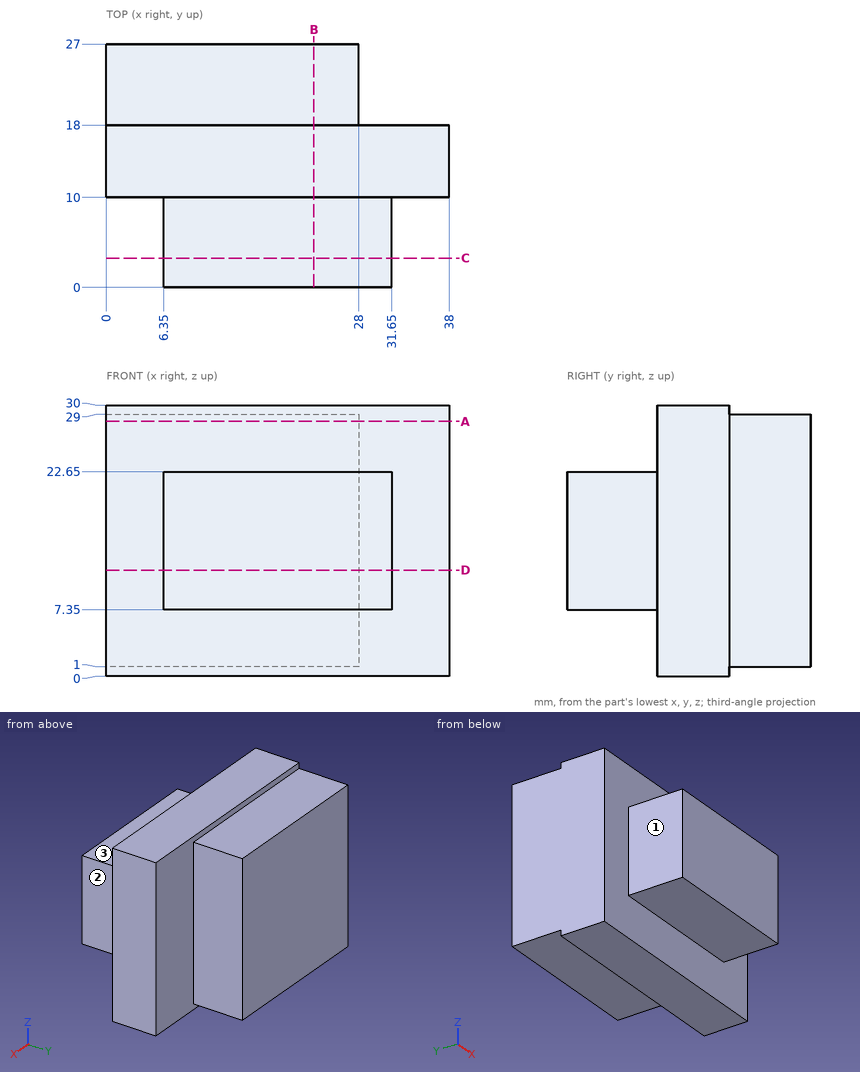
Verification items for this drawing (mm, ordinates from the low corner). A direction names the side the tool comes from. Coordinates: 2 decimals unless noted, no trailing zeros. Order: outer loops, then holes, each group sorted by start corner. A loop starts at its lowest first (then second) coordinate and runs counter-clockwise, first axis right, second up. Notation, with made-up numbers: (-13.5, 35.5) -> (8.5, 35.5) arc R19 ccw to (8.5, 60.5) -> close; hole circle Ø4 at (18, 22.25). An arc over 180 degrees is marked (long way). Answer as CSV lines item,"result". Start each with the question number.
1) Gauge pin test, flat ends, axial feed: pin 1 Ø8 at (y, z) = (3.5, 14) entering from -X; pin 2 Ø5 at (x, y) = (9.5, 23) entering from +Z; pin 3 Ø2 at (x, z) = (19, 4) entering from -Y. Record the tip position at first contact, or that the pin passes through.
2) Cross-section at C-C, the plane y = 3.25. Record the boundary of the cut face in (x, z).
3) Cross-section at B-B, the plane x = 23. Record the boundary of the cut face in (y, z).
4) Cross-section at A-A, the plane z = 28.25. Record the boundary of the cut face in (x, y), then the cut area to 3 significant figures.
5) Cross-section at D-D, the plane z = 11.75. Record the boundary of the cut face in (x, y).
6) Set-up check for the marked faces 1, 2 and 3: record each of +Z, -Z, +X, -X, +Y, -Y from which the full face is reachable in a straight line by a thin tool's end or side.
7) Material ranges on L1, parallel to Y at x = 30, z = 24.75; L2, parallel to Y at x = 15, z = 4.5; L3, parallel to Z at x = 6.5, y = 7.25, recorded low to high. Write a range as [from, to].
Conclusion:
1,pin 1,"stops at x = 6.35"
1,pin 2,"stops at z = 29"
1,pin 3,"stops at y = 10"
2,outline,"(6.35, 7.35) -> (31.65, 7.35) -> (31.65, 22.65) -> (6.35, 22.65) -> close"
3,outline,"(0, 7.35) -> (10, 7.35) -> (10, 0) -> (18, 0) -> (18, 1) -> (27, 1) -> (27, 29) -> (18, 29) -> (18, 30) -> (10, 30) -> (10, 22.65) -> (0, 22.65) -> close"
4,outline,"(0, 10) -> (38, 10) -> (38, 18) -> (28, 18) -> (28, 27) -> (0, 27) -> close"
4,area,"556 mm²"
5,outline,"(0, 10) -> (6.35, 10) -> (6.35, 0) -> (31.65, 0) -> (31.65, 10) -> (38, 10) -> (38, 18) -> (28, 18) -> (28, 27) -> (0, 27) -> close"
6,face 1,"+Z, -Z, -X, -Y"
6,face 2,"+Z, -Z, +X, -Y"
6,face 3,"+Z, +X, -X, -Y"
7,L1,"y = [10, 18]"
7,L2,"y = [10, 27]"
7,L3,"z = [7.35, 22.65]"
